Input: part model. Units: mm. Frame: model coordinates. A direction names the side the tool comes from. Coordinates: 2 decimals unless noted, no trailing zeros. Loops run counter-clockwise (first coordinate to the right, second up) from the corner with the lowest first, then second, coordinate; pieces in that order, holes last. Notation, with made-up numbers: M 0,46 L 32,46 A15 cw 32,72 Z; hole C -34.75,30 d4. An arc over 180 degrees is marked long. Use a Markdown table: item, result. Add a question column.
1. Pin query (flat end, axial travel): pin 1 (5 mm diameter, centred on x = 65, z = -9, fed in from -Y); pin 2 (3.5 mm diameter, centred on x = 25, z = -16, fed in from +Y); pin 3 (2.5 mm diameter, centred on x = -77.5, z = 18, fed in from -Y); pin 4 (2 mm diameter, centred on x = 28, z = 15.5, fed in from +Y). Return the tip coordinate at first contact, or that it passes through.
2. Draft query along Z for faces 1 (the flat face through (-92.5, 2, 1)), 2 (the flat face through (-1, 2, 57.5)), 3 (the flat face through (-87, 2, -53)), 4 (the cylindrical face through (79.57, -2.96, -48.15)). Return one class per face: +Z half, -Z half, draft (parallel to the pull), parting line (faces both ways), or undercut.
3. Line query: L1, parallel to X at y = 1.55, z = 0 (3 decimals); L2, parallel to Z at x = 26.5, y = 3.75; L3, parallel to X at y = -0.5, z = -16. Output: solid intervals per line, ascending. Write a range as [from, to].
4. Section A-A on x = 71.5. Output: boundary loops of the cut face in (y, z), then the cut area to 3 significant figures.
5. Section B-B on z = 28. Output: boundary loops of the cut face in (x, y), then the cut area to 3 significant figures.
6. Set-up query: faces 5 (the flat face through (83, -6, 47)), 6 (the flat face through (24, -3, -14)), 7 (the cylindrical face through (29.2, -1.97, 13.05)). Return all of +Z, -Z, +X, -X, +Y, -Y with unobstructed straight access to the full face (end or side cutting, diameter ignored); none if empty.
```python
from build123d import *

# Parameters (mm, degrees)
SKETCH1_W               = 185
SKETCH1_H               = 115
BOSS_EXTRUDE2_DEPTH     = 5
CUT_EXTRUDE5_DEPTH      = 15
CUT_EXTRUDE5_DEPTH_BACK = 15
SKETCH1_7_OUTSIDE_W     = 230.578
SKETCH1_7_OUTSIDE_H     = 160.578
SKETCH1_7_OUTSIDE_W_2   = 185
SKETCH1_7_OUTSIDE_H_2   = 115
SKETCH1_7_OUTSIDE_R     = 1.375
CHAMFER2_SIZE           = 0.3
SKETCH10_R              = 3
BOSS_EXTRUDE3_DEPTH     = 6
SKETCH11_R              = 4
BOSS_EXTRUDE4_DEPTH     = 4
CUT_EXTRUDE6_DEPTH      = 10
CUT_EXTRUDE6_DEPTH_BACK = 3
SKETCH13_R              = 3.5
CUT_EXTRUDE8_DEPTH      = 7
CUT_EXTRUDE8_DEPTH_BACK = 7
SKETCH14_R              = 1.375
CHAMFER3_SIZE           = 1.625
CHAMFER6_SIZE           = 10
CUT_EXTRUDE9_DEPTH      = 10
CUT_EXTRUDE9_DEPTH_BACK = 10
SKETCH15_W              = 7.1
SKETCH15_H              = 7.1
CHAMFER7_SIZE           = 2


with BuildPart() as part:
    # Sketch1 → Boss-Extrude2 (new body)
    with BuildSketch(Plane(origin=(0, 0, 0), x_dir=(1, 0, 0), z_dir=(0, 1, 0))):
        Rectangle(SKETCH1_W, SKETCH1_H)
    extrude(amount=BOSS_EXTRUDE2_DEPTH)

    # Sketch1<7> outside → Cut-Extrude5 (cut, two sides: drawn at the far end of the back side and taken through both)
    # profile 1 of 9: a face of its own
    with BuildSketch(Plane(origin=(0, 0, 0), x_dir=(1, 0, 0), z_dir=(0, 1, 0)).offset(-CUT_EXTRUDE5_DEPTH_BACK)):
        Rectangle(SKETCH1_7_OUTSIDE_W, SKETCH1_7_OUTSIDE_H)
        Rectangle(SKETCH1_7_OUTSIDE_W_2, SKETCH1_7_OUTSIDE_H_2, mode=Mode.SUBTRACT)
    # profile 2 of 9: a face of its own
    with BuildSketch(Plane(origin=(0, 0, 0), x_dir=(1, 0, 0), z_dir=(0, 1, 0)).offset(-CUT_EXTRUDE5_DEPTH_BACK)):
        with Locations(Location((26.5, 16, 0), (0, 0, 270))):
            Circle(SKETCH1_7_OUTSIDE_R)
    # profile 3 of 9: a face of its own
    with BuildSketch(Plane(origin=(0, 0, 0), x_dir=(1, 0, 0), z_dir=(0, 1, 0)).offset(-CUT_EXTRUDE5_DEPTH_BACK)):
        with Locations(Location((26.5, -16, 0), (0, 0, 270))):
            Circle(SKETCH1_7_OUTSIDE_R)
    # profile 4 of 9: a face of its own
    with BuildSketch(Plane(origin=(0, 0, 0), x_dir=(1, 0, 0), z_dir=(0, 1, 0)).offset(-CUT_EXTRUDE5_DEPTH_BACK)):
        with Locations(Location((-77.5, 36, 0), (0, 0, 270))):
            Circle(SKETCH1_7_OUTSIDE_R)
    # profile 5 of 9: a face of its own
    with BuildSketch(Plane(origin=(0, 0, 0), x_dir=(1, 0, 0), z_dir=(0, 1, 0)).offset(-CUT_EXTRUDE5_DEPTH_BACK)):
        with Locations(Location((-77.5, 18, 0), (0, 0, 270))):
            Circle(SKETCH1_7_OUTSIDE_R)
    # profile 6 of 9: a face of its own
    with BuildSketch(Plane(origin=(0, 0, 0), x_dir=(1, 0, 0), z_dir=(0, 1, 0)).offset(-CUT_EXTRUDE5_DEPTH_BACK)):
        with Locations(Location((-77.5, -18, 0), (0, 0, 270))):
            Circle(SKETCH1_7_OUTSIDE_R)
    # profile 7 of 9: a face of its own
    with BuildSketch(Plane(origin=(0, 0, 0), x_dir=(1, 0, 0), z_dir=(0, 1, 0)).offset(-CUT_EXTRUDE5_DEPTH_BACK)):
        with Locations(Location((-77.5, -36, 0), (0, 0, 270))):
            Circle(SKETCH1_7_OUTSIDE_R)
    # profile 8 of 9: a face of its own
    with BuildSketch(Plane(origin=(0, 0, 0), x_dir=(1, 0, 0), z_dir=(0, 1, 0)).offset(-CUT_EXTRUDE5_DEPTH_BACK)):
        with Locations(Location((-48, 0, 0), (0, 0, 270))):
            Circle(SKETCH1_7_OUTSIDE_R)
    # profile 9 of 9: a face of its own
    with BuildSketch(Plane(origin=(0, 0, 0), x_dir=(1, 0, 0), z_dir=(0, 1, 0)).offset(-CUT_EXTRUDE5_DEPTH_BACK)):
        with Locations(Location((-30, 0, 0), (0, 0, 270))):
            Circle(SKETCH1_7_OUTSIDE_R)
    extrude(amount=CUT_EXTRUDE5_DEPTH + CUT_EXTRUDE5_DEPTH_BACK, mode=Mode.SUBTRACT)

    # Chamfer2
    chamfer2_edges = [part.edges().sort_by_distance(p)[0] for p in [
        (26.5, 5, -17.375),
        (26.5, 5, 14.625),
        (-77.5, 5, -37.375),
        (-77.5, 5, -19.375),
        (-77.5, 5, 16.625),
        (-77.5, 5, 34.625),
        (-48, 5, -1.375),
        (-30, 5, -1.375),
    ]]
    chamfer(chamfer2_edges, length=CHAMFER2_SIZE)

    # Sketch10 → Boss-Extrude3 (add)
    with BuildSketch(Plane(origin=(0, 0, 0), x_dir=(1, 0, 0), z_dir=(0, 1, 0))):
        with Locations(Location((82.5, -47.5, 0), (0, 0, 270))):
            Circle(SKETCH10_R)
        with Locations(Location((82.5, 47.5, 0), (0, 0, 270))):
            Circle(SKETCH10_R)
    extrude(amount=-BOSS_EXTRUDE3_DEPTH)

    # Sketch11 → Boss-Extrude4 (add)
    with BuildSketch(Plane(origin=(0, 0, 0), x_dir=(1, 0, 0), z_dir=(0, 1, 0))):
        with Locations(Location((26.5, -16, 0), (0, 0, 270))):
            Circle(SKETCH11_R)
        with Locations(Location((26.5, 16, 0), (0, 0, 270))):
            Circle(SKETCH11_R)
    extrude(amount=-BOSS_EXTRUDE4_DEPTH)

    # Sketch13 → Cut-Extrude6 (cut, two sides: drawn at the far end of the back side and taken through both)
    with BuildSketch(Plane(origin=(0, 0, 0), x_dir=(1, 0, 0), z_dir=(0, 1, 0)).offset(-CUT_EXTRUDE6_DEPTH_BACK)):
        with Locations(Location((26.5, 16, 0), (0, 0, 270))):
            Circle(SKETCH13_R)
        with Locations(Location((26.5, -16, 0), (0, 0, 270))):
            Circle(SKETCH13_R)
    extrude(amount=CUT_EXTRUDE6_DEPTH + CUT_EXTRUDE6_DEPTH_BACK, mode=Mode.SUBTRACT)

    # Sketch14 → Cut-Extrude8 (cut, two sides: drawn at the far end of the back side and taken through both)
    with BuildSketch(Plane(origin=(0, 0, 0), x_dir=(1, 0, 0), z_dir=(0, 1, 0)).offset(-CUT_EXTRUDE8_DEPTH_BACK)):
        with Locations(Location((26.5, 16, 0), (0, 0, 270))):
            Circle(SKETCH14_R)
        with Locations(Location((26.5, -16, 0), (0, 0, 270))):
            Circle(SKETCH14_R)
    extrude(amount=CUT_EXTRUDE8_DEPTH + CUT_EXTRUDE8_DEPTH_BACK, mode=Mode.SUBTRACT)

    # Chamfer3
    # the kernel refuses this chamfer: 1.625 mm, written as the material it takes off along each edge
    with BuildSketch(Plane(origin=(26.5, -3, 16), x_dir=(0, 0, 1), z_dir=(-1, 0, 0))) as chamfer3_piece_1:
        Polygon((1.375 + CHAMFER3_SIZE, 0), (1.375, -CHAMFER3_SIZE), (1.375, 0), align=None)
    revolve(axis=Axis((26.5, -3, 16), (0, 1, 0)), mode=Mode.SUBTRACT)
    with BuildSketch(Plane(origin=(26.5, -3, -16), x_dir=(0, 0, 1), z_dir=(-1, 0, 0))) as chamfer3_piece_2:
        Polygon((1.375 + CHAMFER3_SIZE, 0), (1.375, -CHAMFER3_SIZE), (1.375, 0), align=None)
    revolve(axis=Axis((26.5, -3, -16), (0, 1, 0)), mode=Mode.SUBTRACT)

    # Chamfer6
    chamfer6_edges = [part.edges().sort_by_distance(p)[0] for p in [
        (-92.5, 2.5, -57.5),
        (92.5, 2.5, -57.5),
        (92.5, 2.5, 57.5),
        (-92.5, 2.5, 57.5),
    ]]
    chamfer(chamfer6_edges, length=CHAMFER6_SIZE)

    # Sketch15 → Cut-Extrude9 (cut, two sides: drawn at the far end of the back side and taken through both)
    with BuildSketch(Plane(origin=(0, 5, 0), x_dir=(1, 0, 0), z_dir=(0, 1, 0)).offset(-CUT_EXTRUDE9_DEPTH_BACK)):
        with Locations((15.5, 0)):
            Rectangle(SKETCH15_W, SKETCH15_H)
    extrude(amount=CUT_EXTRUDE9_DEPTH + CUT_EXTRUDE9_DEPTH_BACK, mode=Mode.SUBTRACT)

    # Chamfer7
    chamfer7_edges = [part.edges().sort_by_distance(p)[0] for p in [
        (19.05, 5, 0),
        (15.5, 5, -3.55),
        (11.95, 5, 0),
        (15.5, 5, 3.55),
    ]]
    chamfer(chamfer7_edges, length=CHAMFER7_SIZE)


solid = part.part
```
Answers below:
| question | item | result |
|---|---|---|
| 1 | pin 1 | stops at y = 0 |
| 1 | pin 2 | stops at y = -3 |
| 1 | pin 3 | passes through |
| 1 | pin 4 | stops at y = -3.42 |
| 2 | face 1 | draft |
| 2 | face 2 | +Z half |
| 2 | face 3 | -Z half |
| 2 | face 4 | undercut |
| 3 | L1 | x = [-92.5, -49.375], [-46.625, -31.375], [-28.625, 11.95], [19.05, 92.5] |
| 3 | L2 | z = [-57.5, -19.5], [-12.5, 12.5], [19.5, 57.5] |
| 3 | L3 | x = [22.5, 23], [30, 30.5] |
| 4 | outline | M 0,-57.5 L 5,-57.5 L 5,57.5 L 0,57.5 Z |
| 4 | area | 575 mm² |
| 5 | outline | M -92.5,0 L 92.5,0 L 92.5,5 L -92.5,5 Z |
| 5 | area | 925 mm² |
| 6 | face 5 | +Z, -Z, +X, -X, -Y |
| 6 | face 6 | +Y |
| 6 | face 7 | -Y |
